Geometry check sheet. Reference: the model listing, model coordinates, mm. Round coordinates to 2 decimals unless told otherwise and drop trailing zeros. Loops run counter-clockwise (first coordinate to the right, second up) from the corner with the lowest first, then second, coordinate; pieces in that order, holes last. Notation, with made-up numbers: M -10,45 L 17,45 A23 cw 17,84 Z; hole C 11,23 d4. An arc over 180 degrees is marked long. Use one line per item in the form item = value. Start each with the question number.
1. Draft check along Z on faces 1 (the cylindrical face through (-0.013, 1.115, -1.216)), 2 (the conical face through (1.49, -3.69, 0.01)), 3 (the conical face through (1.5, 1.8, -3.2)). Enter one of: pulls with the +Z half, pulls with the -Z half, needs draft (parallel to the pull), parting line crosses it, or undercut.
2. Cross-section at A-A (x = -0.45). Record the boundary of the cut face in (y, z).
3. Material ranges on line 1 (Y direction, x = -1, z = 0.75); line 2 (Y direction, x = -0.5, z = 1); line 3 (Z direction, x = 1.1, y = -0.25), recorded low to high.
4. Go/stop test with a flat-tipped pin: pin 1 (1.5 mm diameter, centred on y = -0.5, z = 1, fed in from -X). Record where the tip stops, or that it passes through.
```python
from build123d import *

# Parameters (mm, degrees)
EXTRUDE_M_DEPTH     = 1.6
HOLE_WIZARD_D_D     = 3.3
HOLE_WIZARD_D_DEPTH = 3.2
CHAMFER1_SIZE       = 0.7


with BuildPart() as part:
    # Sketch1 → Extrude m (new body, symmetric)
    with BuildSketch(Plane(origin=(0, 0, 0), x_dir=(0, 0, -1), z_dir=(1, 0, 0))):
        Polygon((0, 4.041451884), (-3.5, 2.020725942), (-3.5, -2.020725942), (0, -4.041451884), (3.5, -2.020725942), (3.5, 2.020725942), align=None)
    extrude(amount=EXTRUDE_M_DEPTH, both=True)

    # Sketch2 → Cut-Revolve1 (revolve, cut)
    with BuildSketch(Plane.XY):
        Polygon((1.6, 4.041451884), (1.287392609, 4.041451884), (1.6, 3.5), align=None)
        Polygon((-1.6, 4.041451884), (-1.6, 3.5), (-1.287392609, 4.041451884), align=None)
    revolve(axis=Axis((0, 0, 0), (1, 0, 0)), mode=Mode.SUBTRACT)

    # Hole Wizard d
    with Locations(Plane(origin=(1.6, 0, 0), x_dir=(0, 0, -1), z_dir=(1, 0, 0))):
        with Locations((0, 0)):
            Hole(HOLE_WIZARD_D_D / 2, depth=HOLE_WIZARD_D_DEPTH)

    # Chamfer1
    chamfer1_edges = [part.edges().sort_by_distance(p)[0] for p in [
        (1.6, 0, -1.65),
        (-1.6, 0, -1.65),
    ]]
    chamfer(chamfer1_edges, length=CHAMFER1_SIZE)


solid = part.part
```
Reported:
q1.face_1 = undercut
q1.face_2 = parting line crosses it
q1.face_3 = pulls with the -Z half
q2.outline = M -4.04,0 L -2.02,-3.5 L 2.02,-3.5 L 4.04,0 L 2.02,3.5 L -2.02,3.5 Z; hole C 0,0 d3.3
q3.line_1 = -3.61 to -1.58, 1.58 to 3.61
q3.line_2 = -3.46 to -1.31, 1.31 to 3.46
q3.line_3 = -3.5 to -1.83, 1.83 to 3.5
q4.pin_1 = -1.12
